from build123d import *

# Parameters (mm, degrees)
SKETCH1_W           = 90
SKETCH1_H           = 71.2
BOSS_EXTRUDE1_DEPTH = 3
SKETCH2_W           = 3
SKETCH2_H           = 2.6
SKETCH2_W_2         = 2.6
SKETCH2_H_2         = 3
BOSS_EXTRUDE2_DEPTH = 4.8
CUT_EXTRUDE1_REACH  = 117.023
SKETCH4_W           = 57
SKETCH4_H           = 60
CUT_EXTRUDE2_REACH  = 117.023
SKETCH5_W           = 14.8
SKETCH5_H           = 8.8
SKETCH5_W_2         = 12
SKETCH5_H_2         = 38
SKETCH6_W           = 1.5
SKETCH6_H           = 9.5
BOSS_EXTRUDE3_DEPTH = 8
BOSS_EXTRUDE4_DEPTH = 9.5


with BuildPart() as part:
    # Sketch1 → Boss-Extrude1 (new body)
    with BuildSketch(Plane(origin=(0, 0, 0), x_dir=(0, 0, -1), z_dir=(1, 0, 0))):
        with Locations((45, 35.6)):
            Rectangle(SKETCH1_W, SKETCH1_H)
    extrude(amount=BOSS_EXTRUDE1_DEPTH)

    # Sketch2 → Boss-Extrude2 (add)
    with BuildSketch(Plane.ZY):
        with Locations((-88.5, 63.7)):
            Rectangle(SKETCH2_W, SKETCH2_H)
        with Locations((-82.5, 69.7)):
            Rectangle(SKETCH2_W_2, SKETCH2_H_2)
        with Locations((-7.5, 69.7)):
            Rectangle(SKETCH2_W_2, SKETCH2_H_2)
        with Locations((-1.5, 63.7)):
            Rectangle(SKETCH2_W, SKETCH2_H)
        with Locations((-1.5, 7.5)):
            Rectangle(SKETCH2_W, SKETCH2_H)
        with Locations((-7.5, 1.5)):
            Rectangle(SKETCH2_W_2, SKETCH2_H_2)
        with Locations((-88.5, 7.5)):
            Rectangle(SKETCH2_W, SKETCH2_H)
        with Locations((-82.5, 1.5)):
            Rectangle(SKETCH2_W_2, SKETCH2_H_2)
    extrude(amount=BOSS_EXTRUDE2_DEPTH)

    # Sketch4 → Cut-Extrude1 (cut, up to next)
    with BuildSketch(Plane(origin=(3, 0, 0), x_dir=(0, 0, -1), z_dir=(1, 0, 0)), mode=Mode.PRIVATE) as cut_extrude1_sk1:
        with Locations((40, 35.6)):
            Rectangle(SKETCH4_W, SKETCH4_H)
    cut_extrude1_tool1 = extrude(cut_extrude1_sk1.sketch, amount=-CUT_EXTRUDE1_REACH, mode=Mode.PRIVATE) & part.part
    add(cut_extrude1_tool1.solids().sort_by_distance((3, 35.6, -40))[0], mode=Mode.SUBTRACT)

    # Sketch5 → Cut-Extrude2 (cut, up to next)
    with BuildSketch(Plane(origin=(3, 0, 0), x_dir=(0, 0, -1), z_dir=(1, 0, 0)), mode=Mode.PRIVATE) as cut_extrude2_sk1:
        with Locations((77.6, 14.4)):
            Rectangle(SKETCH5_W, SKETCH5_H)
    cut_extrude2_tool1 = extrude(cut_extrude2_sk1.sketch, amount=-CUT_EXTRUDE2_REACH, mode=Mode.PRIVATE) & part.part
    # Sketch5 → Cut-Extrude2 (cut, up to next)
    with BuildSketch(Plane(origin=(3, 0, 0), x_dir=(0, 0, -1), z_dir=(1, 0, 0)), mode=Mode.PRIVATE) as cut_extrude2_sk2:
        with Locations((77.75, 42.2)):
            Rectangle(SKETCH5_W_2, SKETCH5_H_2)
    cut_extrude2_tool2 = extrude(cut_extrude2_sk2.sketch, amount=-CUT_EXTRUDE2_REACH, mode=Mode.PRIVATE) & part.part
    add(cut_extrude2_tool1.solids().sort_by_distance((3, 14.4, -77.6))[0], mode=Mode.SUBTRACT)
    add(cut_extrude2_tool2.solids().sort_by_distance((3, 42.2, -77.75))[0], mode=Mode.SUBTRACT)

    # Sketch6 → Boss-Extrude3 (add)
    with BuildSketch(Plane.ZY):
        with Locations((-86.05, 35.6)):
            Rectangle(SKETCH6_W, SKETCH6_H)
    extrude(amount=BOSS_EXTRUDE3_DEPTH)

    # Sketch7 → Boss-Extrude4 (add)
    with BuildSketch(Plane.XZ.offset(-30.85)):
        Polygon((-8, -86.8), (-6.5, -88.3), (-5, -86.8), align=None)
    extrude(amount=-BOSS_EXTRUDE4_DEPTH)


solid = part.part
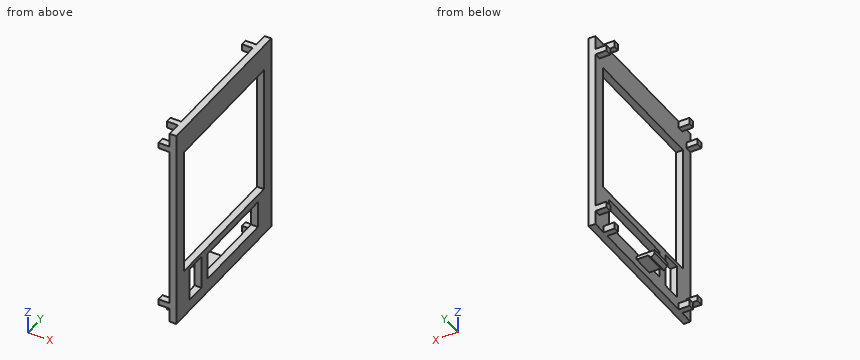
Design review of the part built by this model. Coordinates are the model's own, in mm. Give positions to 0.01 mm unless a question says otherwise; leave off trailing zeros. Loops run counter-clockwise (first coordinate to the right, second up) from the corner with the lowest first, then second, coordinate; pieces in that order, holes last. Notation, with made-up numbers: (12, -1.5) - (67, -1.5) arc R8 ccw to (67, 6.5) - close; hole circle Ø6 at (68, 2). An arc over 180 degrees is marked (long way). Use CSV: the item, a comma, the result in double quotes. Start each with the question number.
1. Add section D-D (y = 15). State the section outline as (x, z) points.
2. Insertion check: P1, Ø0.8, axis at y = 69, z = -7, coming from the -X side; P2, Ø0.9, axis at x = -2, y = 69.5, coming from the +Z side; P3, Ø2.5, axis at x = -1.5, y = 69.5, coming from the -Z side. Each pin has a flat end and moves straight along its axis. Give the tip position at first contact, or say it passes through.
3. Add section C-C (z = -59). State the section outline as (x, y) points, plus the area to 3 significant figures.
4. Add section A-A (y = 55). State the section outline as (x, z) points.
5. Wall thickness on L1, parallel to Z at x = 2.5, y = 48; L2, parallel to Y at x = 1, z = -49; L3, parallel to Z at x = 1, y = 8.5: over which ranges is each line inside the solid? List them lowest first.
6. Add section B-B (z = -82.5). State the section outline as (x, y) points, plus the area to 3 significant figures.
Results found:
1,outline,"(0, -90) - (3, -90) - (3, -85) - (0, -85) - close; (0, -70.2) - (3, -70.2) - (3, -68.5) - (0, -68.5) - close; (0, -11.5) - (3, -11.5) - (3, 0) - (0, 0) - close"
2,P1,"stops at x = -4.8"
2,P2,"stops at z = -6.2"
2,P3,"stops at z = -83.8"
3,outline,"(0, 0) - (3, 0) - (3, 5.6) - (0, 5.6) - close; (0, 65.6) - (3, 65.6) - (3, 71.2) - (0, 71.2) - close"
3,area,"33.6 mm²"
4,outline,"(0, -90) - (3, -90) - (3, -83.75) - (0, -83.75) - close; (0, -71.75) - (3, -71.75) - (3, -68.5) - (0, -68.5) - close; (0, -11.5) - (3, -11.5) - (3, 0) - (0, 0) - close"
5,L1,"z = -90 to -83.75, -71.75 to -68.5, -11.5 to 0"
5,L2,"y = 0 to 5.6, 65.6 to 71.2"
5,L3,"z = -90 to -68.5, -11.5 to 0"
6,outline,"(-4.8, 0) - (3, 0) - (3, 10) - (0, 10) - (0, 3) - (-4.8, 3) - close; (-4.8, 68.2) - (0, 68.2) - (0, 61.2) - (3, 61.2) - (3, 71.2) - (-4.8, 71.2) - close; (0, 18.8) - (3, 18.8) - (3, 23.2) - (0, 23.2) - close"
6,area,"102 mm²"
